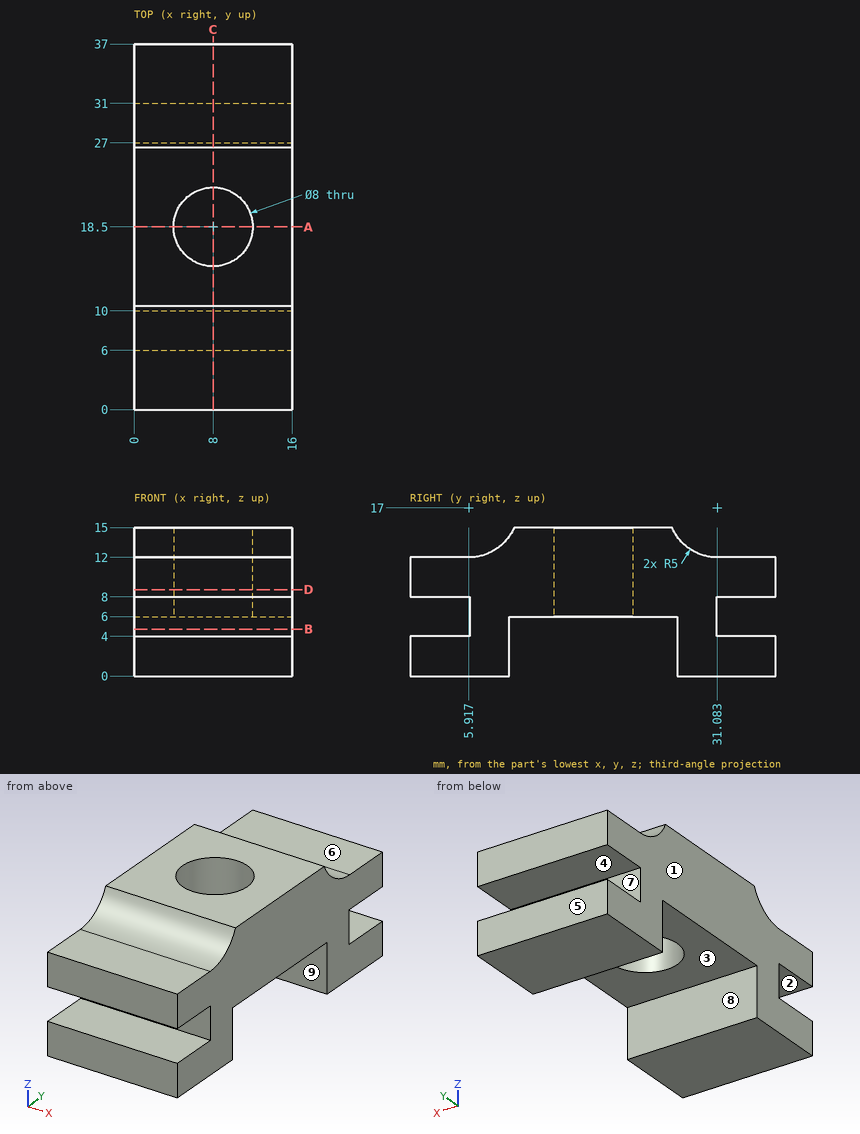
Geometry: see drawing. Coordinates: mm, zero at the bounding-box minimum. A direction names the side the tool comes from. Give positions to 0.01 mm unless a question says otherwise; leave off trailing zeros. Order: outer loops, then holes, each group sorted by start corner. A loop starts at its lowest first (then second) coordinate and runs counter-clockwise, first axis right, second up. Notation, with made-up numbers: (24.5, 34) -> (67.5, 34) arc R27 ccw to (67.5, 73) -> close; hole circle Ø6 at (34.5, 31). An arc over 180 degrees is marked (long way). Write each question's results on one line, items separated by ' | '. Start each with the question number.
1) Set-up query: the marked faces 1, 2, 3, 4 and 5. Return all of +Z, -Z, +X, -X, +Y, -Y with unobstructed straight access to the full face (end or side cutting, diameter ignored); none if empty.
2) Line query: line 1 (Z direction, x = 14.75, y = 34); line 2 (Y direction, x = 8, z = 8.5); line 3 (Z direction, x = 2.25, y = 16). Output: solid intervals per line, ascending. Write a range as from..to.
3) Section A-A (y = 18.5). Return loops of the section in (x, z).
4) Section D-D (z = 8.75). Return loops of the section in (x, y).
5) Section B-B (z = 4.75). Return loops of the section in (x, y).
6) Section C-C (x = 8). Return loops of the section in (y, z), then the cut area to 3 significant figures.
7) Draft query along Y for the marked faces 6, 7, 8 and 9. Return one class per face: pulls with the +Y half, pulls with the -Y half, needs draft (parallel to the pull), parting line crosses it, or undercut.
8) First-contact query: pin 1 (8 mm diameter, centred on x = 10, y = 19.5, fed in from -Z); pin 2 (1.8 mm diameter, centred on x = 9, y = 4, fed in from +Z); pin 3 (2 mm diameter, centred on x = 12.5, y = 6, fed in from +Z). Flat tips, straight axial feed; report the tip coordinate or a pass-through.
Calculated:
1) face 1: +Z, -Z, -X, +Y, -Y | face 2: +X, -X, -Y | face 3: -Z, +X, -X | face 4: +X, -X, +Y | face 5: +Z, -Z, +X, -X, +Y
2) line 1: 0..4, 8..12 | line 2: 0..14.5, 22.5..37 | line 3: 6..15
3) outline: (0, 6) -> (4, 6) -> (4, 15) -> (0, 15) -> close; (12, 6) -> (16, 6) -> (16, 15) -> (12, 15) -> close
4) outline: (0, 0) -> (16, 0) -> (16, 37) -> (0, 37) -> close; hole circle Ø8 at (8, 18.5)
5) outline: (0, 6) -> (16, 6) -> (16, 10) -> (0, 10) -> close; (0, 27) -> (16, 27) -> (16, 31) -> (0, 31) -> close
6) outline: (0, 0) -> (10, 0) -> (10, 6) -> (14.5, 6) -> (14.5, 15) -> (10.5, 15) arc R5 cw to (5.92, 12) -> (0, 12) -> (0, 8) -> (6, 8) -> (6, 4) -> (0, 4) -> close; (22.5, 6) -> (27, 6) -> (27, 0) -> (37, 0) -> (37, 4) -> (31, 4) -> (31, 8) -> (37, 8) -> (37, 12) -> (31.08, 12) arc R5 cw to (26.5, 15) -> (22.5, 15) -> close | area: 278 mm2
7) face 6: needs draft | face 7: pulls with the +Y half | face 8: undercut | face 9: undercut
8) pin 1: z = 6 | pin 2: z = 12 | pin 3: z = 12.12
